Autodesk Inventor part; units mm, degrees
ref_plane "YZ Plane" through (0, 0, 0) normal (1, 0, 0) x (0, 1, 0)
ref_plane "XZ Plane" through (0, 0, 0) normal (0, 1, 0) x (-1, 0, 0)
ref_plane "XY Plane" through (0, 0, 0) normal (0, 0, 1) x (1, 0, 0)
sketch "スケッチ1" plane through (0, 0, 0) normal (0, 0, 1) x (1, 0, 0)
  line L0 (-59.5, -21.75) -> (59.5, -21.75) construction
  line L1 (59.5, -21.75) -> (59.5, 21.75) construction
  line L2 (59.5, 21.75) -> (-59.5, 21.75) construction
  line L3 (-59.5, 21.75) -> (-59.5, -21.75) construction
  line L4 (-59.5, -21.75) -> (59.5, 21.75) construction
  line L5 (59.5, -21.75) -> (-59.5, 21.75) construction
  line L6 (-54.5, -16.75) -> (54.5, -16.75) construction
  line L7 (54.5, -16.75) -> (54.5, 16.75) construction
  line L8 (54.5, 16.75) -> (-54.5, 16.75) construction
  line L9 (-54.5, 16.75) -> (-54.5, -16.75) construction
  line L10 (-54.5, -16.75) -> (54.5, 16.75) construction
  line L11 (54.5, -16.75) -> (-54.5, 16.75) construction
  line L12 (-33.05, 11.05) -> (-27.95, 11.05)
  line L13 (-27.95, 11.05) -> (-27.95, -4.05)
  line L14 (-27.95, -4.05) -> (-33.05, -4.05)
  line L15 (-33.05, -4.05) -> (-33.05, 11.05)
  line L16 (-28, 11) -> (-33, 11) construction
  line L17 (-33, 11) -> (-33, -4) construction
  line L18 (-33, -4) -> (-28, -4) construction
  line L19 (-28, -4) -> (-28, 11) construction
  line L20 (-30.5, 11) -> (-30.5, -4) construction
  line L21 (-33, 21) -> (-28, 21) construction
  line L22 (-28, 21) -> (-28, -14) construction
  line L23 (-28, -14) -> (-33, -14) construction
  line L24 (-33, -14) -> (-33, 21) construction
  circle A0 centre (-30.5, 17) radius 1.55
  circle A1 centre (-30.5, -10) radius 1.55
  circle A2 centre (-33.05, 10) radius 1.05
  circle A3 centre (-27.95, 10) radius 1.05
  circle A4 centre (-33.05, -3) radius 1.05
  circle A5 centre (-27.95, -3) radius 1.05
  line L25 (0, 0) -> (0, 16.75) construction
  line L26 (0, 0) -> (54.5, 0) construction
  circle A6 centre (30.5, 17) radius 1.55
  circle A7 centre (30.5, -10) radius 1.55
  circle A8 centre (27.95, 10) radius 1.05
  circle A9 centre (33.05, 10) radius 1.05
  circle A10 centre (27.95, -3) radius 1.05
  circle A11 centre (33.05, -3) radius 1.05
  line L27 (33.05, 11.05) -> (27.95, 11.05)
  line L28 (27.95, 11.05) -> (27.95, -4.05)
  line L29 (27.95, -4.05) -> (33.05, -4.05)
  line L30 (33.05, -4.05) -> (33.05, 11.05)
  line L31 (-59.5, 11.75) -> (-62.5, 11.75)
  line L32 (-62.5, 11.75) -> (-62.5, -11.75)
  line L33 (-62.5, -11.75) -> (-59.5, -11.75)
  line L34 (-59.5, 13.85) -> (-59.5, 21.75)
  line L35 (-59.5, 21.75) -> (-21.6, 21.75)
  line L36 (-19.5, 21.75) -> (-19.5, 26.75)
  line L37 (-19.5, 26.75) -> (19.5, 26.75)
  line L38 (19.5, 26.75) -> (19.5, 21.75)
  line L39 (21.6, 21.75) -> (59.5, 21.75)
  line L40 (59.5, 21.75) -> (59.5, 13.85)
  line L41 (59.5, 11.75) -> (62.5, 11.75)
  line L42 (62.5, 11.75) -> (62.5, -11.75)
  line L43 (62.5, -11.75) -> (59.5, -11.75)
  line L44 (-59.5, -13.85) -> (-59.5, -21.75)
  line L45 (-59.5, -21.75) -> (59.5, -21.75)
  line L46 (59.5, -21.75) -> (59.5, -13.85)
  arc A12 (-59.5, 11.75) -> (-59.5, 13.85) centre (-59.5, 12.8) ccw
  arc A13 (-59.5, -13.85) -> (-59.5, -11.75) centre (-59.5, -12.8) ccw
  line L47 (0, 0) -> (-54.5, 0) construction
  arc A14 (59.5, -11.75) -> (59.5, -13.85) centre (59.5, -12.8) ccw
  arc A15 (59.5, 13.85) -> (59.5, 11.75) centre (59.5, 12.8) ccw
  arc A16 (-21.6, 21.75) -> (-19.5, 21.75) centre (-20.55, 21.75) ccw
  arc A17 (19.5, 21.75) -> (21.6, 21.75) centre (20.55, 21.75) ccw
  line L48 (-56.8855, 19.3) -> (-54.5, 19.3) construction
  line L49 (-54.5, 19.3) -> (-54.5, 16.2) construction
  line L50 (-54.5, 16.2) -> (-56.8855, 16.2) construction
  line L51 (-56.8855, 16.2) -> (-56.8855, 19.3) construction
  line L52 (-54.5, 17.75) -> (-56.8855, 17.75) construction
  line L53 (-53.05, 22.7202) -> (-49.95, 22.7202) construction
  line L54 (-49.95, 22.7202) -> (-49.95, 16.75) construction
  line L55 (-49.95, 16.75) -> (-53.05, 16.75) construction
  line L56 (-53.05, 16.75) -> (-53.05, 22.7202) construction
  line L57 (-51.5, 22.7202) -> (-51.5, 16.75) construction
  point P0 (-30.5, -14)
  dimension "d10" = 2.1
  dimension "d0" = 33.5
  dimension "d1" = 5
  dimension "d2" = 109
  dimension "d3" = 5
  dimension "d4" = 0.05
  dimension "d5" = 35
  dimension "d6" = 27
  dimension "d7" = 5
  dimension "d11" = 33
  dimension "d12" = 3.1
  dimension "d13" = 1.05
  dimension "d14" = 3
  dimension "d15" = 4
  dimension "d16" = 3.1
  dimension "d17" = 10
  dimension "d18" = 5
  dimension "d19" = 8
  dimension "d20" = 5
  dimension "d21" = 40
  dimension "d22" = 5
  dimension "d50" = 4
  dimension "d51" = 10
  dimension "d52" = 17
  dimension "d53" = 10
extrude "押し出し1" add sketch "スケッチ1" along normal blind 5
sketch "スケッチ2" plane through (0, 0, 5) normal (0, 0, 1) x (1, 0, 0)
  circle A0 centre (30.5, -10) radius 1.55
  circle A1 centre (30.5, 17) radius 1.55
  circle A2 centre (-30.5, -10) radius 1.55
  circle A3 centre (-30.5, 17) radius 1.55
  point P0 (0, 0)
hole "穴1" at (-30.5, 17, 5) at (-30.5, -10, 5) at (30.5, 17, 5) at (30.5, -10, 5) direction (0, 0, -1) diameter 6 depth 3
sketch "スケッチ3" plane through (59.5, -21.75, 0) normal (1, 0, 0) x (0, 0, -1)
  line L0 (0, 0) -> (-5, 0)
  line L1 (0, 43.5) -> (-5, 43.5)
  point P0 (0, 21.75)
  point P1 (-2.5, 4)
  point P2 (-2.5, 39.5)
  point P3 (-2.5, 0)
  dimension "d32" = 4
  dimension "d33" = 4
hole "穴2" at (59.5, -17.75, 2.5) at (59.5, 17.75, 2.5) direction (-1, 0, 0) diameter 2.459 depth 2.5
mirror "ミラー1" about plane through (0, 0, 0) normal (1, 0, 0) of "穴2"
sketch "スケッチ5" plane through (0, 0, 5) normal (0, 0, 1) x (1, 0, 0)
  line L0 (27.95, -1.95) -> (27.95, 8.95)
  line L1 (-33.05, -1.95) -> (-33.05, 8.95)
  line L2 (-27.95, 8.95) -> (-27.95, -1.95)
  line L3 (-59.5, -21.75) -> (59.5, -21.75)
  line L4 (19.5, 26.75) -> (-19.5, 26.75)
  line L5 (-21.6, 21.75) -> (-59.5, 21.75)
  line L6 (-59.5, 21.75) -> (-59.5, 13.85)
  line L7 (-52.5, 14.75) -> (-38, 14.75)
  line L8 (-38, 14.75) -> (-38, -14.75)
  line L9 (-38, -14.75) -> (-52.5, -14.75)
  line L10 (-52.5, -14.75) -> (-52.5, 14.75)
  line L11 (38, 14.75) -> (52.5, 14.75)
  line L12 (52.5, 14.75) -> (52.5, -14.75)
  line L13 (52.5, -14.75) -> (38, -14.75)
  line L14 (38, -14.75) -> (38, 14.75)
  line L15 (-23, 16.75) -> (-23, -9.0978)
  line L16 (-23, -9.0978) -> (20.2083, 16.75)
  line L17 (20.2083, 16.75) -> (-23, 16.75)
  line L18 (23, 9.0978) -> (23, -16.75)
  line L19 (23, -16.75) -> (-20.2083, -16.75)
  line L20 (-20.2083, -16.75) -> (23, 9.0978)
  line L21 (-33, 9.2736) -> (-28, 9.2736) construction
  line L22 (-28, 9.2736) -> (-28, -5.1442) construction
  line L23 (-28, -5.1442) -> (-33, -5.1442) construction
  line L24 (-33, -5.1442) -> (-33, 9.2736) construction
  line L25 (0, 0) -> (0, 26.75) construction
  line L26 (28, 10.3975) -> (29.3974, 10.3975) construction
  line L27 (29.3974, 10.3975) -> (29.3974, -4.5864) construction
  line L28 (29.3974, -4.5864) -> (28, -4.5864) construction
  line L29 (28, -4.5864) -> (28, 10.3975) construction
  line L30 (28, 16.75) -> (-28, -16.75) construction
  line L31 (-28, 16.75) -> (28, 16.75) construction
  line L32 (28, 16.75) -> (28, -16.75) construction
  line L33 (28, -16.75) -> (-28, -16.75) construction
  line L34 (-28, -16.75) -> (-28, 16.75) construction
  line L35 (59.5, 21.75) -> (21.6, 21.75)
  dimension "d54" = 7
  dimension "d55" = 7
  dimension "d56" = 7
  dimension "d57" = 0.05
  dimension "d58" = 5
  dimension "d59" = 0.05
  dimension "d60" = 5
  dimension "d62" = 5
  dimension "d63" = 0.05
  dimension "d64" = 8
  dimension "d68" = 5
extrude "押し出し2" cut sketch "スケッチ5" against normal blind 10
fillet "フィレット1" radius 3 14 edges at (-38, 14.75, 2.5) (-52.5, 14.75, 2.5) (-52.5, -14.75, 2.5) (-38, -14.75, 2.5) (-23, -9.0978, 2.5) (-23, 16.75, 2.5) (20.2083, 16.75, 2.5) (23, 9.0978, 2.5) (-20.2083, -16.75, 2.5) (23, -16.75, 2.5) (38, -14.75, 2.5) (52.5, -14.75, 2.5) (52.5, 14.75, 2.5) (38, 14.75, 2.5)
equation "\"d20\" = d18"
equation "\"d53\" = d51"
equation "\"d56\" = d55"
equation "\"d59\" = d57"
equation "\"d60\" = d58"
properties part number "コックピット_サブフレーム_1_3" material "アセタール樹脂、黒"
Model file for the job. Use its own axes, mm. A direction names the side the tool comes from. Coordinates: 2 decimals unless noted, no trailing zeros. Order: outer loops, then holes, each group sorted by start corner. A loop starts at its lowest first (then second) coordinate and runs counter-clockwise, first axis right, second up. Notation, with made-up numbers: (21, 7) -> (58, 7) arc R20 ccw to (58, 46) -> close; hole circle Ø10 at (79.5, 52.5). An arc over 180 degrees is marked (long way). Return JSON: item names as keys, results as strings. Group by question number.
Item 1: Tool access for faces 4 (the cylindrical face through (-51.64, 13.85, 2.46)), 5 (the cylindrical face through (-58.45, 12.82, 2.46)), 6 (the flat face through (61, 11.75, 2)): list every direction of +Z, -Z, +X, -X, +Y, -Y with a clear straight run to the whole face (end or side of a thin tool).
Item 2: Saw through at D-D on y = -10. State how many separate pieces and enclosed holes the cut face has, then the cut area to 3 significant figures.
Item 3: Wall check: line 1 along Y through (x, z) = (30.5, 3.6); line 2 along Y through (x, z) = (42, 0.8); line 3 along X through (y, z) = (17, 1). Give the ranges that are in metal, low to high. Write a range as [from, to].
Item 4: Pull direction X, two halves, no side cores. Call faces 1 (the cylindrical face through (58.23, 16.53, 2.66)), 2 (the cylindrical face through (-34.1, -3, 2.5)), 3 (the flat face through (59.5, 19, 1)): pulls with the +X half, pulls with the -X half, needs draft (parallel to the pull), parting line crosses it, or undercut.
Item 5: Saw through at B-B on y = 0.5. Write the cut outline in (x, z), then the cut area to 3 significant figures.
Item 6: Saw through at A-A on x = 30.5. Write the cut outline in (y, z), then the cut area to 3 significant figures.
Item 7: Saw through at C-C on x = -7. Write the cut outline in (y, z).
Item 8: Flat gauge pins, fed straight in: P1, Ø1.5, axis at y = -17.75, z = 2.5, coming from the -X side; P2, Ø2.5, axis at y = -18, z = 2, coming from the -X side; P3, Ø1.5, axis at y = 16, z = 3.5, coming from the +X side. Where does each tip first touch, or does it go through?
Values found:
{
 "1": {"face 4": "+Z, -Z", "face 5": "+Z, -Z, -X", "face 6": "+Z, -Z, +X, +Y"},
 "2": {"separate pieces": "6", "enclosed holes": "0", "area": "272 mm2"},
 "3": {"line 1": "y = [-21.75, -13], [-7, -4.05], [11.05, 14], [20, 21.75]", "line 2": "y = [-21.75, -14.75], [14.75, 21.75]", "line 3": "x = [-59.5, -32.05], [-28.95, 28.95], [32.05, 59.5]"},
 "4": {"face 1": "needs draft", "face 2": "undercut", "face 3": "pulls with the +X half"},
 "5": {"outline": "(-62.5, 0) -> (-52.5, 0) -> (-52.5, 5) -> (-62.5, 5) -> close; (-38, 0) -> (-33.05, 0) -> (-33.05, 5) -> (-38, 5) -> close; (-27.95, 0) -> (-23, 0) -> (-23, 5) -> (-27.95, 5) -> close; (-6.96, 0) -> (8.63, 0) -> (8.63, 5) -> (-6.96, 5) -> close; (23, 0) -> (27.95, 0) -> (27.95, 5) -> (23, 5) -> close; (33.05, 0) -> (38, 0) -> (38, 5) -> (33.05, 5) -> close; (52.5, 0) -> (62.5, 0) -> (62.5, 5) -> (52.5, 5) -> close", "area": "277 mm2"},
 "6": {"outline": "(-21.75, 0) -> (-11.55, 0) -> (-11.55, 2) -> (-13, 2) -> (-13, 5) -> (-21.75, 5) -> close; (-8.45, 0) -> (-4.05, 0) -> (-4.05, 5) -> (-7, 5) -> (-7, 2) -> (-8.45, 2) -> close; (11.05, 0) -> (15.45, 0) -> (15.45, 2) -> (14, 2) -> (14, 5) -> (11.05, 5) -> close; (18.55, 0) -> (21.75, 0) -> (21.75, 5) -> (20, 5) -> (20, 2) -> (18.55, 2) -> close", "area": "93.6 mm2"},
 "7": {"outline": "(-21.75, 0) -> (-16.75, 0) -> (-16.75, 5) -> (-21.75, 5) -> close; (-8.85, 0) -> (0.47, 0) -> (0.47, 5) -> (-8.85, 5) -> close; (16.75, 0) -> (26.75, 0) -> (26.75, 5) -> (16.75, 5) -> close"},
 "8": {"P1": "stops at x = -57", "P2": "stops at x = -59.5", "P3": "stops at x = 59.5"}
}
